Here's how the part is built. I have some questions about the finished solid (model axes, mm). A direction names the side the tool comes from. Give positions to 0.01 mm unless a question says otherwise; leave off trailing zeros. Loops run counter-clockwise (first coordinate to the right, second up) from the corner with the lowest first, then second, coordinate; pieces in that order, holes last. Notation, with made-up numbers: (49, -17) -> (99, -17) arc R28 cw to (99, 1) -> close; hole circle Ø6 at (1, 11). An arc over 180 degrees is marked (long way). Answer in a Markdown table with one row per item. Add a question column.
Item 1: If we section it at C-C (y = 0): Write out the boundary of the cut face in (x, z), then the cut area to 4 significant figures.
Item 2: If we section it at A-A (x = -4.5): Write out the boundary of the cut face in (y, z), then the cut area to 3 significant figures.
Item 3: If I drill on line 1 (Y direction, x = 13, z = 11.5) (3 decimals); line 2 (Y direction, x = -5.5, z = 3); line 3 (Z direction, x = 5.5, y = -3.25), over which ranges is the centre line in solid material (lowest first)?
Item 4: If we section it at D-D (x = 16): Write out the boundary of the cut face in (y, z) (3 decimals).
Item 5: If we section it at B-B (z = 11.5): Write out the boundary of the cut face in (x, y) (3 decimals).
Item 6: We'd pull the mould along X, two halves only. Please class faces 1 (the face through (-13, 0, 2)), 2 (the face through (-5, 7, 8)), 3 (the face through (-12, 0, 3.5)), 4 (the face through (19.248, -8.287, 7.605)): released by +X, released by -X, zero draft, split by the parting line, or undercut.
Item 7: Which directions (+Z, -Z, +X, -X, +Y, -Y) give clear straight access to the entire face, cutting with the end or side of a thin tool? Please do faces 5 (the face through (6.409, -6.076, 8.409)), 6 (the face through (-11, -5.5, 9)), 7 (the face through (16.8, -0.1, 2.1)), 8 (the face through (3, -9, 7)).
Item 8: For P1, Ø2.5, axis at y = 1.5, z = 5.5, coming from the -X side; P2, Ø1.5, axis at x = -11.5, y = -1.5, coming from the +Z side; P3, Ø1.5, axis at x = -11.5, z = 10.5, coming from the +Y side, each with a flat end and sliding along its axis, tell me the tip position at first contact or that it passes through.
Autodesk Fusion 360 part; units mm, degrees
sketch "Sketch1" plane through (0, 0, 0) normal (0, 0, 1) x (1, 0, 0)
  line L0 (0, 0) -> (0, 7)
  line L1 (0, 0) -> (0, -7)
  line L2 (0, 0) -> (20, 0)
  line L3 (20, 0) -> (20, -5.125)
  line L4 (20, 0) -> (20, 5.125)
  line L5 (0, 0) -> (13, 0)
  line L6 (20, 5.125) -> (13, 5.125)
  line L7 (13, 5.125) -> (13, -5.125)
  line L8 (13, -5.125) -> (20, -5.125)
  line L9 (20, -5.125) -> (20, 5.125)
  line L10 (0, 7) -> (13, 5.125)
  line L11 (0, -7) -> (13, -5.125)
  line L12 (0, 7) -> (-10, 7)
  line L13 (-10, 7) -> (-10, -7)
  line L14 (-10, -7) -> (0, -7)
  line L15 (0, -7) -> (0, 7)
  line L16 (-10, 0) -> (-10, 5.5)
  line L17 (-10, 0) -> (-10, -5.5)
  line L18 (20, -9) -> (0, -9)
  line L19 (0, -9) -> (0, 9)
  line L20 (0, 9) -> (20, 9)
  line L21 (20, 9) -> (20, -9)
  line L22 (20, -9) -> (0, 9) construction
  line L23 (0, -9) -> (20, 9) construction
  line L24 (-13, -9) -> (13, -9)
  line L25 (13, -9) -> (13, 9)
  line L26 (13, 9) -> (-13, 9)
  line L27 (-13, 9) -> (-13, -9)
  line L28 (-13, -9) -> (13, 9) construction
  line L29 (13, -9) -> (-13, 9) construction
  line L30 (-10, 5.5) -> (-13, 5.5)
  line L31 (-10, -5.5) -> (-13, -5.5)
  point P0 (10, 0)
  dimension "d1" = 7
  dimension "d2" = 5.125
  dimension "d3" = 5.125
  dimension "d4" = 13
  dimension "d5" = 5.5
  dimension "d6" = 5.5
extrude "Extrude1" add sketch "Sketch1" along normal blind 15 contours L10 L19 L20 L25 L26 | L12 L13 L19 L26 L27 L30 | L13 L14 L19 L24 L27 L31 | L11 L18 L19 L24 L25 | L6 L20 L21 L25 | L8 L18 L21 L25 makes body 1 at (-2, -9, 5) makes body 2 at (9, 9, 5)
extrude "Extrude2" add sketch "Sketch1" along normal blind 2 contours L0 L1 L12 L13 L14 L15 L16 L17 L19 | L1 L2 L5 L7 L11 L15 L19 L25 | L0 L2 L5 L7 L10 L15 L19 L25 | L2 L4 L6 L7 L9 L21 L25 | L2 L3 L7 L8 L9 L21 L25 bodies 1 2
extrude "Extrude3" add sketch "Sketch1" along normal blind 3.5 contours L13 L16 L17 L27 L30 L31 bodies 1
sketch "Sketch2" plane through (20, 0, 0) normal (1, 0, 0) x (0, 1, 0)
  line L0 (-9, 0) -> (9, 0)
  line L1 (9, 0) -> (9, 15)
  line L2 (9, 15) -> (5.125, 15)
  line L3 (5.125, 15) -> (5.125, 2)
  line L4 (5.125, 2) -> (-5.125, 2)
  line L5 (-5.125, 2) -> (-5.125, 15)
  line L6 (-5.125, 15) -> (-9, 15)
  line L7 (-9, 15) -> (-9, 0)
  line L8 (0, 2) -> (0, 7.1)
  circle A0 centre (0, 7.1) radius 5
  line L9 (-5, 7.1) -> (-5.125, 7.1)
  line L10 (5, 7.1) -> (5.125, 7.1)
  dimension "d13" = 5.1
  dimension "d14" = 10
extrude "Extrude4" add sketch "Sketch2" against normal blind 6.5 contours L4 L5 L8 A0 L9 | L3 L4 L8 A0 L10 bodies 1
chamfer "Chamfer1" distance 0.1 angle 45 2 edges at (16.75, -5, 7.1) (16.75, 5, 7.1) on bodies 1
fillet "Fillet1" radius 2.5 4 edges at (-13, -9, 7.5) (20, -9, 7.5) (-13, 9, 7.5) (20, 9, 7.5) on bodies 1
Recorded:
| question | item | result |
|---|---|---|
| 1 | outline | (-13, 0) -> (20, 0) -> (20, 2.1) -> (13.5, 2.1) -> (13.5, 2) -> (-10, 2) -> (-10, 3.5) -> (-13, 3.5) -> close |
| 1 | area | 71.15 mm^2 |
| 2 | outline | (-9, 0) -> (9, 0) -> (9, 15) -> (7, 15) -> (7, 2) -> (-7, 2) -> (-7, 15) -> (-9, 15) -> close |
| 2 | area | 88.0 mm^2 |
| 3 | line 1 | y = -9 to -5.125, 5.125 to 9 |
| 3 | line 2 | y = -9 to -7, 7 to 9 |
| 3 | line 3 | z = 0 to 2 |
| 4 | outline | (-9, 0) -> (9, 0) -> (9, 15) -> (5.125, 15) -> (5.125, 7.1) -> (5.1, 7.1) -> (4.999, 7) arc R5 cw to (-4.999, 7) -> (-5.1, 7.1) -> (-5.125, 7.1) -> (-5.125, 15) -> (-9, 15) -> close |
| 5 | outline | (-13, -6.5) arc R2.5 ccw to (-10.5, -9) -> (17.5, -9) arc R2.5 ccw to (20, -6.5) -> (20, -5.125) -> (13, -5.125) -> (0, -7) -> (-10, -7) -> (-10, -5.5) -> (-13, -5.5) -> close; (-13, 5.5) -> (-10, 5.5) -> (-10, 7) -> (0, 7) -> (13, 5.125) -> (20, 5.125) -> (20, 6.5) arc R2.5 ccw to (17.5, 9) -> (-10.5, 9) arc R2.5 ccw to (-13, 6.5) -> close |
| 6 | face 1 | released by -X |
| 6 | face 2 | undercut |
| 6 | face 3 | zero draft |
| 6 | face 4 | released by +X |
| 7 | face 5 | +Z |
| 7 | face 6 | +Z, -X |
| 7 | face 7 | +Z, +X |
| 7 | face 8 | +Z, -Z, +X, -X, -Y |
| 8 | P1 | passes through |
| 8 | P2 | stops at z = 3.5 |
| 8 | P3 | stops at y = 8.99 |
